Geometry check sheet. Reference: drawing and pictorial views, mm from the part's lowest x, y, z. Coordinates: 2 decimals unless noted, no trailing zeros. Write each loop counter-clockwise with the first axis right and the second up, starting at its lowest first coordinate (ties: lowest second). Pieces come first, ordered by that corner, then holes. Notation, with made-up numbers: (30, -9.75) -> (46, -9.75) arc R11 ccw to (46, -5.75) -> close; hole circle Ø10 at (30.25, 13.5). An arc over 180 degrees is marked (long way). Answer in a Markdown table with one row per item.
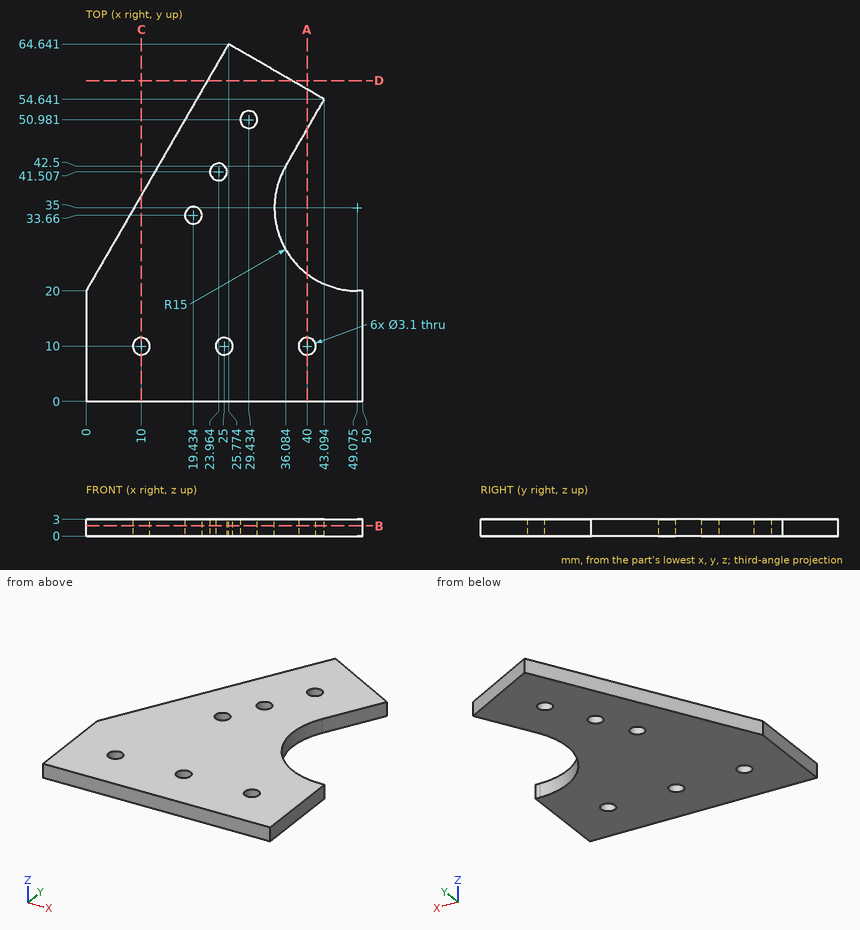
1. Section check B-B, the plane z = 1.85. State how many separate pieces and enclosed holes the cut face has, plus the area to 3 significant figures.
Geometry says:
| item | result |
|---|---|
| separate pieces | 1 |
| enclosed holes | 6 |
| area | 2,020 mm^2 |
2. Section check D-D, the plane y = 58. Record the boundary of the cut face in (x, z), plus the area to 3 significant figures.
Geometry says:
| item | result |
|---|---|
| outline | (21.94, 0) -> (37.28, 0) -> (37.28, 3) -> (21.94, 3) -> close |
| area | 46.0 mm^2 |
3. Section check C-C, the plane x = 10. Record the boundary of the cut face in (y, z).
Geometry says:
| item | result |
|---|---|
| outline | (0, 0) -> (8.45, 0) -> (8.45, 3) -> (0, 3) -> close; (11.55, 0) -> (37.32, 0) -> (37.32, 3) -> (11.55, 3) -> close |
4. Depth check by flat-ended pin: P1, Ø1.5, axis at x = 37, y = 44, coming from the +Z side; P2, Ø1, axis at x = 50, z = 2, coming from the +Y side; P3, Ø1.5, axis at y = 37, z = 0.5, coming from the +X side; P4, Ø3, axis at x = 29.43, y = 50.98, coming from the -Z side. Enter the tip coordinate at first touch or a pass-through.
Geometry says:
| item | result |
|---|---|
| P1 | z = 3 |
| P2 | y = 20 |
| P3 | x = 34.33 |
| P4 | through |
5. Thickness scan on line 1 (X direction, y = 11, z = 0.8) (1 decimal); line 2 (X direction, y = 9.5, z = 1.9); line 3 (Y direction, x = 10, z = 1.1). Record the ranges inside material, lowest first. Write a range as from..to.
Geometry says:
| item | result |
|---|---|
| line 1 | 0..8.8, 11.2..23.8, 26.2..38.8, 41.2..50 |
| line 2 | 0..8.53, 11.47..23.53, 26.47..38.53, 41.47..50 |
| line 3 | 0..8.45, 11.55..37.32 |
6. Section check A-A, the plane x = 40. Record the boundary of the cut face in (y, z).
Geometry says:
| item | result |
|---|---|
| outline | (0, 0) -> (8.45, 0) -> (8.45, 3) -> (0, 3) -> close; (11.55, 0) -> (23.06, 0) -> (23.06, 3) -> (11.55, 3) -> close; (49.28, 0) -> (56.43, 0) -> (56.43, 3) -> (49.28, 3) -> close |
